Verification items for the finished model (mm, model axes). A direction names the side the tool comes from. Give positions to 0.01 mm unless a question says otherwise; leave off trailing zeros. Write each loop counter-clockwise with the first axis right and the second up, starting at its lowest first coordinate (ties: lowest second). Pieces come first, ordered by that corner, then holes. Notation, with made-up numbers: (-8.75, 59.5) -> (29.25, 59.5) arc R25 cw to (29.25, 96.5) -> close; hole circle Ø7 at (78.25, -21). An arc over 180 degrees is marked (long way). Answer as CSV lines item,"result". Start each with the question number.
1) Material ranges on L1, parallel to X at y = 3, z = 14; L2, parallel to Y at x = -15, z = 12.5, recorded low to high.
2) Sectioned sample at B-B on y = 7. Record the cut outline in (x, z).
3) Tool access check on faces 4 (the flat face through (0, 18.5, 14)), 5 (the flat face through (16, 17, 4)), 6 (the flat face through (17, -16, 24)), 7 (the cylindrical face through (-8.474, 18.852, 14.14)). Record the directions out of +Z, -Z, +X, -X, +Y, -Y that give a thin tool (end or side, any length) a straight path to the whole face; none if there is none.
4) Sectioned sample at D-D on z = 24.5. Record the cut outline in (x, y), and give its area (3 significant figures).
5) Mould release check, pull along X, two halves, no side actions. Record for faces 1 (the flat face through (-10, 17, 0)), 2 (the cylindrical face through (-18.852, -8.474, 14.14)), 3 (the flat face through (-13.3, -13.2, 14.2)): released by +X, released by -X, zero draft, split by the parting line, or undercut.
6) Gauge pin test, flat end, axial feed: pin 1 Ø2 at (y, z) = (14.5, 10) entering from -X. Record the tip position at first contact, or that the pin passes through.
Autodesk Inventor part; units mm, degrees
ref_plane "YZ Plane" through (0, 0, 0) normal (1, 0, 0) x (0, 1, 0)
ref_plane "XZ Plane" through (0, 0, 0) normal (0, 1, 0) x (-1, 0, 0)
ref_plane "XY Plane" through (0, 0, 0) normal (0, 0, 1) x (1, 0, 0)
sketch "Sketch1" plane through (0, 0, 0) normal (0, 0, 1) x (1, 0, 0)
  line L0 (19, -19) -> (-19, -19)
  line L1 (-19, -19) -> (-19, 19)
  line L2 (-19, 19) -> (19, 19)
  line L3 (19, 19) -> (19, -19)
  line L4 (19, -19) -> (-19, 19) construction
  line L5 (-19, -19) -> (19, 19) construction
  point P0 (0, 0)
  dimension "d0" = 38
  dimension "d1" = 38
extrude "Extrusion1" add sketch "Sketch1" along normal blind 4
sketch "Sketch2" plane through (0, 0, 4) normal (0, 0, 1) x (1, 0, 0)
  line L0 (19, 19) -> (-19, 19)
  line L1 (-19, 19) -> (-19, -19)
  line L2 (8.547, -19) -> (-8.547, -19)
  line L3 (-19, -8.547) -> (-19, 8.547)
  line L4 (-8.547, 19) -> (8.547, 19)
  line L5 (19, 8.547) -> (19, -8.547)
  line L6 (19, -19) -> (-19, 19) construction
  line L7 (-19, -19) -> (19, 19) construction
  line L8 (19, 6.0309) -> (19, -12.9361)
  line L9 (-19, 8.547) -> (-8.547, 19)
  line L10 (8.547, 19) -> (19, 8.547)
  line L11 (19, -8.547) -> (8.547, -19)
  line L12 (-8.547, -19) -> (-19, -8.547)
  point P0 (0, 0)
  dimension "d16" = 38
  dimension "d17" = 38
  dimension "d18" = 10.453
  dimension "d19" = 10.453
  dimension "d20" = 10.453
  dimension "d21" = 10.453
  dimension "d22" = 10.453
  dimension "d23" = 10.453
  dimension "d24" = 10.453
  dimension "d25" = 10.453
extrude "Extrusion2" add sketch "Sketch2" along normal blind 20 contours L10 L5 L11 L2 L12 L1 L9 L0
sketch "Sketch3" plane through (0, 0, 24) normal (0, 0, 1) x (1, 0, 0)
  line L0 (19, 19) -> (-19, 19)
  line L1 (19, -19) -> (-19, -19)
  line L2 (-19, -19) -> (-19, 19)
  line L3 (-19, 19) -> (19, 19)
  line L4 (19, 19) -> (19, -19)
  line L5 (19, -19) -> (-19, 19) construction
  line L6 (-19, -19) -> (19, 19) construction
  point P0 (0, 0)
extrude "Extrusion3" add sketch "Sketch3" along normal blind 4
sketch "Sketch5" plane through (0, 0, 28) normal (0, 0, 1) x (1, 0, 0)
  line L0 (8, -18.5) -> (-8, -18.5)
  line L1 (-18.5, -8) -> (-18.5, 8)
  line L2 (-8, 18.5) -> (8, 18.5)
  line L3 (18.5, 8) -> (18.5, -8)
  line L4 (18.5, -18.5) -> (-18.5, 18.5) construction
  line L5 (-18.5, -18.5) -> (18.5, 18.5) construction
  line L6 (-18.5, 8) -> (-8, 18.5)
  line L7 (8, 18.5) -> (18.5, 8)
  line L8 (18.5, -8) -> (8, -18.5)
  line L9 (-18.5, -8) -> (-8, -18.5)
  point P0 (0, 0)
  dimension "d27" = 37
  dimension "d28" = 37
  dimension "d29" = 10.5
  dimension "d30" = 10.5
  dimension "d31" = 10.5
  dimension "d32" = 10.5
  dimension "d33" = 10.5
  dimension "d34" = 10.5
  dimension "d35" = 10.5
  dimension "d36" = 10.5
extrude "Extrusion5" cut sketch "Sketch5" against normal blind 28
fillet "Fillet2" radius 2 16 edges at (19, 19, 26) (19, 19, 2) (-19, 19, 26) (-19, 19, 2) (-19, -19, 26) (-19, -19, 2) (19, -19, 26) (19, -19, 2) (19, -8.547, 14) (8.547, -19, 14) (-8.547, -19, 14) (-19, -8.547, 14) (-19, 8.547, 14) (-8.547, 19, 14) (8.547, 19, 14) (19, 8.547, 14)
sketch "Sketch6" plane through (0, 0, 28) normal (0, 0, 1) x (1, 0, 0)
  line L0 (-15, -15) -> (15, -15) construction
  line L1 (15, -15) -> (15, 15) construction
  line L2 (15, 15) -> (-15, 15) construction
  line L3 (-15, 15) -> (-15, -15) construction
  line L4 (-15, -15) -> (15, 15) construction
  line L5 (15, -15) -> (-15, 15) construction
  circle A0 centre (15, 15) radius 1.85
  circle A1 centre (15, -15) radius 1.85
  circle A2 centre (-15, -15) radius 1.85
  circle A3 centre (-15, 15) radius 1.85
  point P0 (0, 0)
  dimension "d40" = 30
  dimension "d41" = 30
  dimension "d42" = 3.7
  dimension "d43" = 3.7
  dimension "d44" = 3.7
  dimension "d45" = 3.7
extrude "Extrusion6" cut sketch "Sketch6" against normal blind 28
equation "\"d19\" = d18"
equation "\"d20\" = d18"
equation "\"d21\" = d20"
equation "\"d22\" = d18"
equation "\"d23\" = d22"
equation "\"d24\" = d18"
equation "\"d25\" = d24"
equation "\"d30\" = d29"
equation "\"d31\" = d29"
equation "\"d32\" = d31"
equation "\"d33\" = d29"
equation "\"d34\" = d33"
equation "\"d35\" = d29"
equation "\"d36\" = d35"
properties part number "fan"
Ans:
1,L1,"x = -19 to -18.5, 18.5 to 19"
1,L2,"y = -12.55 to -11.5, 11.5 to 12.55"
2,outline,"(-19, 0) -> (-18.5, 0) -> (-18.5, 28) -> (-19, 28) -> close; (18.5, 0) -> (19, 0) -> (19, 28) -> (18.5, 28) -> close"
3,face 4,"+Z, -Z"
3,face 5,"+X, +Y"
3,face 6,"+X, -Y"
3,face 7,"-X, +Y"
4,outline,"(-19, -17) arc R2 ccw to (-17, -19) -> (17, -19) arc R2 ccw to (19, -17) -> (19, 17) arc R2 ccw to (17, 19) -> (-17, 19) arc R2 ccw to (-19, 17) -> close; hole (-18.5, -8) -> (-8, -18.5) -> (8, -18.5) -> (18.5, -8) -> (18.5, 8) -> (8, 18.5) -> (-8, 18.5) -> (-18.5, 8) -> close; hole circle Ø3.7 at (-15, -15); hole circle Ø3.7 at (-15, 15); hole circle Ø3.7 at (15, -15); hole circle Ø3.7 at (15, 15)"
4,area,"249 mm²"
5,face 1,"zero draft"
5,face 2,"released by -X"
5,face 3,"undercut"
6,pin 1,"stops at x = -13.92"
